Verification items for the finished model (mm, model axes). A direction names the side the tool comes from. Round coordinates to 2 decimals unless told otherwise and drop trailing zeros. Loops run counter-clockwise (first coordinate to the right, second up) from the corner with the lowest first, then second, coordinate; pieces in that order, holes last. Notation, with made-up numbers: (40, 48) -> (75, 48) arc R23 ccw to (75, 81) -> close; hole circle Ø2 at (32.5, 42). An arc over 180 degrees is marked (long way). Use a Markdown table: item, result. Add a question column.
```python
from build123d import *

# Parameters (mm, degrees)
SKICA1_W                 = 50
SKICA1_H                 = 50
P_IDAT_VYSUNUT_M2_DEPTH  = 3
SKICA5_W                 = 50
SKICA5_H                 = 5
ODEBRAT_VYSUNUT_M3_DEPTH = 1
P_IDAT_VYSUNUT_M9_DEPTH  = 15
SKICA17_R                = 2
ODEBRAT_VYSUNUT_M8_DEPTH = 4


with BuildPart() as part:
    # Skica1 → Přidat vysunutím2 (new body)
    with BuildSketch(Plane.XY):
        Rectangle(SKICA1_W, SKICA1_H)
    extrude(amount=P_IDAT_VYSUNUT_M2_DEPTH)

    # Skica5 → Odebrat vysunutím3 (cut)
    with BuildSketch(Plane(origin=(0, 0, 0), x_dir=(-1, 0, 0), z_dir=(0, 0, -1))):
        Rectangle(SKICA5_W, SKICA5_H)
    extrude(amount=-ODEBRAT_VYSUNUT_M3_DEPTH, mode=Mode.SUBTRACT)

    # Skica14 → Přidat vysunutím9 (add)
    with BuildSketch(Plane.XY.offset(3)):
        Polygon((25, 25), (-25, 25), (-25, -25), (-24, -25), (-24, 24), (24, 24), (24, -25), (25, -25), align=None)
    extrude(amount=P_IDAT_VYSUNUT_M9_DEPTH)

    # Skica17 → Odebrat vysunutím8 (cut)
    with BuildSketch(Plane(origin=(0, 0, 1), x_dir=(-1, 0, 0), z_dir=(0, 0, -1))):
        with Locations((-16, 0)):
            Circle(SKICA17_R)
        with Locations((16, 0)):
            Circle(SKICA17_R)
    extrude(amount=-ODEBRAT_VYSUNUT_M8_DEPTH, mode=Mode.SUBTRACT)


solid = part.part
```
1) Release check for a two-part mould opening along X. For faces 1 (the face through (0, 24, 10)), 2 (the face through (0, -14, 0)), 3 (the face through (25, 0, 9)), 4 (the face through (24, 0, 10)) record: released by +X, released by -X, zero draft, split by the parting line, or undercut.
2) Sectioned sample at A-A on x = -16. Enter the section's corners in (y, z), then the cut area to 3 significant figures.
3) Sectioned sample at D-D on z = 9.25. Enter the section's corners in (x, y).
4) Sectioned sample at B-B on y = 0. Enter the section's corners in (x, z).
5) Thickness scan on line 1 (X direction, y = -3.5, z = 4.75); line 2 (Y direction, x = -16, z = 1.7); line 3 (Z direction, x = 8.5, y = -14.5). Record the ranges inside material, lowest first.
6) Go/stop test with flat-tipped pins: pin 1 (2.5 mm diameter, centred on x = 16, y = 0, fed in from +Z); pin 2 (1.5 mm diameter, centred on x = 8.5, y = 0, fed in from -Z); pin 3 (5 mm diameter, centred on x = -12, y = -14.5, fed in from -Z). Record where each tip stops, or that it passes through.
7) Access from +Z, -Z, +X, -X, +Y, -Y to the whole of each face (thin tool, end or side, straight path). Record for faces 5 (the face through (-4, -25, 2)), 6 (the face through (0, 0, 3)), 7 (the face through (0, 0, 1)).
8) Sectioned sample at C-C on y = -5. Enter the section's corners in (x, z), then the cut area to 3 significant figures.
Geometry results:
| question | item | result |
|---|---|---|
| 1 | face 1 | undercut |
| 1 | face 2 | zero draft |
| 1 | face 3 | released by +X |
| 1 | face 4 | undercut |
| 2 | outline | (-25, 0) -> (-2.5, 0) -> (-2.5, 1) -> (-2, 1) -> (-2, 3) -> (-25, 3) -> close; (2, 1) -> (2.5, 1) -> (2.5, 0) -> (25, 0) -> (25, 18) -> (24, 18) -> (24, 3) -> (2, 3) -> close |
| 2 | area | 152 mm^2 |
| 3 | outline | (-25, -25) -> (-24, -25) -> (-24, 24) -> (24, 24) -> (24, -25) -> (25, -25) -> (25, 25) -> (-25, 25) -> close |
| 4 | outline | (-25, 1) -> (-18, 1) -> (-18, 3) -> (-24, 3) -> (-24, 18) -> (-25, 18) -> close; (-14, 1) -> (14, 1) -> (14, 3) -> (-14, 3) -> close; (18, 1) -> (25, 1) -> (25, 18) -> (24, 18) -> (24, 3) -> (18, 3) -> close |
| 5 | line 1 | -25 to -24, 24 to 25 |
| 5 | line 2 | -25 to -2, 2 to 25 |
| 5 | line 3 | 0 to 3 |
| 6 | pin 1 | through |
| 6 | pin 2 | z = 1 |
| 6 | pin 3 | z = 0 |
| 7 | face 5 | +Z, -Z, +X, -X, -Y |
| 7 | face 6 | +Z, -Y |
| 7 | face 7 | -Z, +X, -X |
| 8 | outline | (-25, 0) -> (25, 0) -> (25, 18) -> (24, 18) -> (24, 3) -> (-24, 3) -> (-24, 18) -> (-25, 18) -> close |
| 8 | area | 180 mm^2 |
